Can you work these out from the model? Positions are in its coordinate system, mm. A direction names the side the tool comes from. Give positions to 0.01 mm unless a question says otherwise; leave off trailing zeros. Write each loop counter-clockwise with the first axis right and the second up, starting at its lowest first coordinate (ties: lowest second). Pieces come first, ordered by that corner, then holes.
```python
from build123d import *

# Parameters (mm, degrees)
F3_DEPTH = 41.798657


with BuildPart() as f1:
    # F0 (on Front) → F1 (revolve)
    with BuildSketch(Plane.XZ):
        with BuildLine():
            ThreePointArc((-27, -30), (-38.886788, -13.87103), (-53.330974, 0.01439))
            ThreePointArc((-53.330974, 0.01439), (-59.670879, 4.754114), (-66, 0))
            Line((-66, 0), (-66, -4.929408))
            Line((-66, -4.929408), (-67.825363, -4.929408))
            ThreePointArc((-67.825363, -4.929408), (-69.314377, -1.439596), (-72.824865, 0))
            Line((-72.824865, 0), (-88.9, 0))
            Line((-88.9, 0), (-88.9, -41.797657))
            Line((-88.9, -41.797657), (0, -41.797657))
            Line((0, -41.797657), (0, -20))
            ThreePointArc((0, -20), (-13.47012, -22.5747), (-25, -30))
            Line((-25, -30), (-27, -30))
        make_face()
    revolve(axis=Axis((0, 0, -11.485694), (0, 0, -1)))

    # F2 (on face) → F3 (cut, through all)
    with BuildSketch(Plane.XY):
        Polygon((-59.565999, 82.5), (-33.120386, 82.5), (33.120386, 82.5), (63.941218, 82.5), (-2.141983, 104.541838), align=None)
        Polygon((33.120386, -82.5), (-33.120386, -82.5), (-49.083836, -82.5), (6.972946, -111.715175), (56.649286, -82.5), align=None)
    extrude(amount=-F3_DEPTH, mode=Mode.SUBTRACT)


solid = f1.part
```
1) For faces 4 (the face through (0, 82.5, -21)), 5 (the face through (15, -65, -4.929)), which set-ups out of +Z, -Z, +X, -X, +Y, -Y let a thin tool reach every point of the face, with its end or its side?
Values follow:
face 4: +Z, -Z, +X, -X, +Y
face 5: +Z
2) Suppose I cut it at B-B on z = -10. Write out the boundary of the cut face in (x, y).
Values follow:
outline: (-33.12, -82.5) - (33.12, -82.5) arc R88.9 ccw to (33.12, 82.5) - (-33.12, 82.5) arc R88.9 ccw to start; hole circle Ø84.88 at (0, 0)
3) Suppose I cut it at A-A on z = -27.5. State how many separate pieces and enclosed holes the cut face has, plus the area to 3 significant figures.
Values follow:
separate pieces: 2
enclosed holes: 1
area: 23,200 mm2
4) For pin 1 Ø2 at (y, z) = (40.5, -36.5) entering from -X; pin 2 Ø16 at (x, y) = (-6, 4.5) entering from +Z; pin 3 Ø1.5 at (y, z) = (-29.5, -19.5) entering from +X, each with a flat end and sliding along its axis, tell me the tip position at first contact or that it passes through.
Values follow:
pin 1: stops at x = -79.64
pin 2: stops at z = -20
pin 3: stops at x = 84.12
5) If we mould it in two halves opening along X, with no side actions, what happens to faces 1 (the face through (24, -8, -30)), 2 (the face through (1, 1, -41.798)), 3 (the face through (-88.888, -1.48, -21.191))? For each: +X half, -X half, draft (parallel to the pull), parting line (faces both ways), or undercut.
Values follow:
face 1: undercut
face 2: draft
face 3: -X half
6) Please list where these lines run through material, in increasing order: L1, parallel to Y at x = -12, z = -0.5; L2, parallel to Y at x = -57, z = -2; L3, parallel to Z at x = 17, y = -70.5.
Values follow:
L1: y = -82.5 to -69.62, -64.9 to -51.32, 51.32 to 64.9, 69.62 to 82.5
L2: y = -68.22 to -38.57, -33.27 to 33.27, 38.57 to 68.22
L3: z = -41.8 to -0.01
